CAD build for the part. Positions are in the model's coordinates, mm. A direction names the side the tool comes from. Coordinates: 2 decimals unless noted, no trailing zeros. Write each loop counter-clockwise with the first axis right and the second up, starting at its lowest first coordinate (ties: lowest second). Pieces come first, ordered by that corner, then holes.
Autodesk Inventor part; units mm, degrees
ref_plane "YZ Plane" through (0, 0, 0) normal (1, 0, 0) x (0, 1, 0)
ref_plane "XZ Plane" through (0, 0, 0) normal (0, 1, 0) x (-1, 0, 0)
ref_plane "XY Plane" through (0, 0, 0) normal (0, 0, 1) x (1, 0, 0)
sketch "Sketch1" plane through (0, 0, 0) normal (0, 0, 1) x (1, 0, 0)
  line L0 (0, 1.7321) -> (1.5, 0.866)
  line L1 (1.5, 0.866) -> (1.5, -0.866)
  line L2 (1.5, -0.866) -> (0, -1.7321)
  line L3 (0, -1.7321) -> (-1.5, -0.866)
  line L4 (-1.5, -0.866) -> (-1.5, 0.866)
  line L5 (-1.5, 0.866) -> (0, 1.7321)
  point P0 (0, 0)
  point P1 (0, 0)
  dimension "d0" = 3
extrude "Extrusion1" add sketch "Sketch1" along normal blind 5
sketch "Sketch2" plane through (0, 0, 5) normal (0, 0, 1) x (1, 0, 0)
  circle A0 centre (0, 0) radius 1
  dimension "d3" = 2
extrude "Extrusion2" cut sketch "Sketch2" against normal blind 3
sketch "Sketch3" plane through (0, 0, 0) normal (0, 0, -1) x (-1, 0, 0)
  circle A0 centre (0, 0) radius 1
extrude "Extrusion3" add sketch "Sketch3" along normal blind 3
thread "Thread1"
thread "Thread2"
properties part number "M2_5mm_standoff"
Item 1: Saw through at B-B, the plane x = -0.2. Write the cut outline in (y, z), and give its area (3 significant figures).
Item 2: Wall check: line 1 along X through (y, z) = (-0.5, 3.5); line 2 along Z through (x, y) = (1, 0.35); line 3 along Z through (x, y) = (-0.7, -0.45). Give the ranges that are in metal, low to high.
Item 3: Saw through at A-A, the plane y = 0. Write the cut outline in (x, z), and give its area (3 significant figures).
Item 4: Two-plate mould, pull along X, no slides. Class faces 1 (the flat face through (0.74, 1.305, 2.465)), 2 (the flat face through (-0.4, -1.1, 0)), 3 (the flat face through (0, 0, 2)): +X half, -X half, draft (parallel to the pull), parting line (faces both ways), or undercut.
Item 5: Which spindle directions (+Z, -Z, +X, -X, +Y, -Y) get a long thin tool onto all of the face, cutting with end or side? Do faces 4 (the flat face through (-0.4, -1.1, 5)), 5 (the cylindrical face through (0, 1, -1)), 6 (the cylindrical face through (0, -1, 4)). Say none if no direction does.
Item 6: Saw through at D-D, the plane x = -1.2. Write the cut outline in (y, z).
Item 7: Flat gauge pins, fed straight in: pin 1 Ø1.5 at (x, y) = (-1, 1.5) entering from -Z; pin 2 Ø1.8 at (x, y) = (0, 0) entering from +Z. Where does each tip first touch, or does it go through?
Item 8: Saw through at C-C, the plane z = 0.5. Write the cut outline in (x, y), and give its area (3 significant figures).
Working result:
1. outline: (-1.62, 0) - (-0.98, 0) - (-0.98, -3) - (0.98, -3) - (0.98, 0) - (1.62, 0) - (1.62, 5) - (0.98, 5) - (0.98, 2) - (-0.98, 2) - (-0.98, 5) - (-1.62, 5) - close
1. area: 16.2 mm2
2. line 1: x = -1.5 to -0.87, 0.87 to 1.5
2. line 2: z = 0 to 5
2. line 3: z = -3 to 2
3. outline: (-1.5, 0) - (-1, 0) - (-1, -3) - (1, -3) - (1, 0) - (1.5, 0) - (1.5, 5) - (1, 5) - (1, 2) - (-1, 2) - (-1, 5) - (-1.5, 5) - close
3. area: 15.0 mm2
4. face 1: +X half
4. face 2: draft
4. face 3: undercut
5. face 4: +Z, +X, -X, +Y, -Y
5. face 5: -Z
5. face 6: +Z
6. outline: (-1.04, 0) - (1.04, 0) - (1.04, 5) - (-1.04, 5) - close
7. pin 1: stops at z = 0
7. pin 2: stops at z = 2
8. outline: (-1.5, -0.87) - (0, -1.73) - (1.5, -0.87) - (1.5, 0.87) - (0, 1.73) - (-1.5, 0.87) - close
8. area: 7.79 mm2
